Part model, mm, in its own coordinate system. Face numbers are marked on the shaded views. Give positions to 0.01 mm unless a question says otherwise; leave off trailing zeros. Order: outer loops, then holes, each group sorted by start corner. A loop starts at its lowest first (then second) coordinate and runs counter-clockwise, first axis right, second up. Notation, with made-up numbers: (15.5, -32) -> (68.5, -32) arc R16 cw to (68.5, -3) -> close; hole circle Ø4 at (75, 40.25). An arc over 180 degrees is marked (long way). Write item = value, one per line. Start each with the question number.
(1) Saw through at B-B, the plane y = 1. List the corners of the cut face in (x, z), then the cut area to 3 significant figures.
(2) Saw through at C-C, the plane z = 2.4. List the corners of the cut face in (x, y), then the cut area to 3 significant figures.
(3) Flat gauge pin, fed straight in: pin 1 (2 mm diameter, centred on x = -2, y = -3, fed in from -Z). Where does the tip first touch, or does it go through?
(4) Two-plate mould, pull along Y, no slides. Class the marked faces 1, 2 and 3: pulls with the +Y half, pulls with the -Y half, needs draft (parallel to the pull), parting line crosses it, or undercut.
(5) Probe line 1 along Y through (x, z) = (0, 1.15); line 2 along X through (y, z) = (-1, 1.65); line 3 along X through (y, z) = (-9.5, 1.85). List the from-to ranges inside material, lowest first. Write a range as from..to.
(6) Saw through at D-D, the plane y = -18. List the corners of the cut face in (x, z).
(7) Saw through at A-A, the plane x = 0. List the corners of the cut face in (y, z), then the cut area to 3 significant figures.
from build123d import *

# Parameters (mm, degrees)
BOSS_EXTRUDE1_DEPTH = 3
SKETCH2_R           = 2.5
CUT_EXTRUDE1_DEPTH  = 34.51119216
SKETCH3_R           = 1.5
CUT_EXTRUDE2_DEPTH  = 34.51119216


with BuildPart() as part:
    # Sketch1 → Boss-Extrude1 (new body)
    with BuildSketch(Plane.XY):
        with BuildLine():
            Line((-5, 0), (-3, -30))
            ThreePointArc((-3, -30), (0, -33), (3, -30))
            Line((3, -30), (5, 0))
            ThreePointArc((5, 0), (0, 5), (-5, 0))
        make_face()
    extrude(amount=BOSS_EXTRUDE1_DEPTH)

    # Sketch2 → Cut-Extrude1 (cut, through all)
    with BuildSketch(Plane.XY.offset(3)):
        Circle(SKETCH2_R)
    extrude(amount=-CUT_EXTRUDE1_DEPTH, mode=Mode.SUBTRACT)

    # Sketch3 → Cut-Extrude2 (cut, through all)
    with BuildSketch(Plane.XY.offset(3)):
        with Locations((0, -29.973330892)):
            Circle(SKETCH3_R)
    extrude(amount=-CUT_EXTRUDE2_DEPTH, mode=Mode.SUBTRACT)


solid = part.part
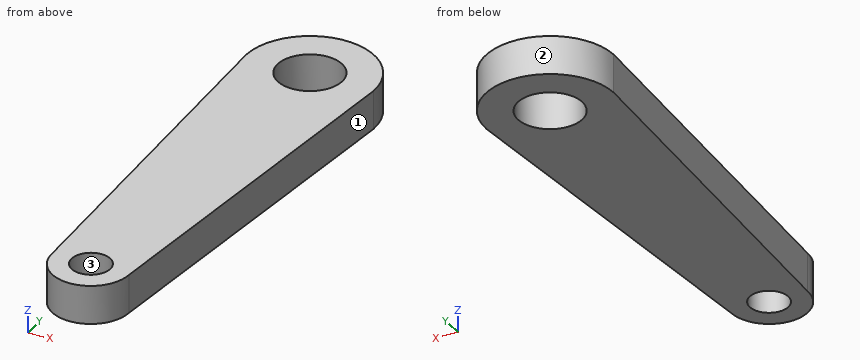
Results list:
q1.outline = (-4.9, 0) -> (-2.29, 0) -> (-2.29, 3) -> (-4.9, 3) -> close; (2.29, 0) -> (4.9, 0) -> (4.9, 3) -> (2.29, 3) -> close
q1.area = 15.6 mm^2
q2.outline = (-5, 0) -> (-3, -30) arc R3 ccw to (3, -30) -> (5, 0) arc R5 ccw to start; hole circle Ø5 at (0, 0); hole circle Ø3 at (0, -29.97)
q2.area = 267 mm^2
q3.pin_1 = 0
q4.face_1 = pulls with the -Y half
q4.face_2 = pulls with the +Y half
q4.face_3 = undercut
q5.line_1 = -33..-31.47, -28.47..-2.5, 2.5..5
q5.line_2 = -4.93..-2.29, 2.29..4.93
q5.line_3 = -4.37..4.37
q6.outline = (-3.8, 0) -> (3.8, 0) -> (3.8, 3) -> (-3.8, 3) -> close
q7.outline = (-33, 0) -> (-31.47, 0) -> (-31.47, 3) -> (-33, 3) -> close; (-28.47, 0) -> (-2.5, 0) -> (-2.5, 3) -> (-28.47, 3) -> close; (2.5, 0) -> (5, 0) -> (5, 3) -> (2.5, 3) -> close
q7.area = 90.0 mm^2
